```python
from build123d import *

# Parameters (mm, degrees)
F1_DEPTH  = 3.5
F2_W      = 30
F2_H      = 3
F3_DEPTH  = 14.5
F4_W      = 30
F4_H      = 3
F5_DEPTH  = 15
F6_W      = 3
F6_H      = 75
F7_DEPTH  = 14.5
F8_W      = 3
F8_H      = 75
F9_DEPTH  = 14.5
F10_W     = 3
F10_H     = 75
F11_DEPTH = 3
F12_W     = 3
F12_H     = 75
F13_DEPTH = 3
F14_R     = 2
F15_R     = 2
F16_R     = 2
F18_D     = 4.4


with BuildPart() as f1:
    # F0 (on Front) → F1 (new body)
    with BuildSketch(Plane.XZ):
        Polygon((15, 82.5), (-15, 82.5), (-15, 37.5), (-39, 37.5), (-39, -37.5), (-15, -37.5), (-15, -82.5), (15, -82.5), (15, -37.5), (39, -37.5), (39, 37.5), (15, 37.5), align=None)
    extrude(amount=F1_DEPTH)

    # F2 (on face) → F3 (join)
    with BuildSketch(Plane.XZ.offset(3.5)):
        with Locations((0, -81)):
            Rectangle(F2_W, F2_H)
    extrude(amount=F3_DEPTH)

    # F4 (on face) → F5 (join)
    with BuildSketch(Plane.XY.offset(-79.5)):
        with Locations((0, -16.5)):
            Rectangle(F4_W, F4_H)
    extrude(amount=F5_DEPTH)

    # F6 (on face) → F7 (join)
    with BuildSketch(Plane.XZ.offset(3.5)):
        with Locations((-37.5, 0)):
            Rectangle(F6_W, F6_H)
    extrude(amount=F7_DEPTH)

    # F8 (on face) → F9 (join)
    with BuildSketch(Plane.XZ.offset(3.5)):
        with Locations((37.5, 0)):
            Rectangle(F8_W, F8_H)
    extrude(amount=F9_DEPTH)

    # F10 (on face) → F11 (join)
    with BuildSketch(Plane.YZ.offset(-36)):
        with Locations((-16.5, 0)):
            Rectangle(F10_W, F10_H)
    extrude(amount=F11_DEPTH)

    # F12 (on face) → F13 (join)
    with BuildSketch(Plane(origin=(36, 0, 0), x_dir=(0, -1, 0), z_dir=(-1, 0, 0))):
        with Locations((16.5, 0)):
            Rectangle(F12_W, F12_H)
    extrude(amount=F13_DEPTH)

    # F14
    f14_edges = [f1.edges().sort_by_distance(p)[0] for p in [
        (39, -18, 0),
    ]]
    fillet(f14_edges, radius=F14_R)

    # F15
    f15_edges = [f1.edges().sort_by_distance(p)[0] for p in [
        (-39, -18, 0),
    ]]
    fillet(f15_edges, radius=F15_R)

    # F16
    f16_edges = [f1.edges().sort_by_distance(p)[0] for p in [
        (0, -18, -82.5),
    ]]
    fillet(f16_edges, radius=F16_R)

    # F18 (through all)
    with Locations(Plane.XZ.offset(3.5)):
        with Locations((0, 74.796483)):
            Hole(F18_D / 2)


solid = f1.part
```
Model file for the job. Use its own axes, mm. A direction names the side the tool comes from. Coordinates: 2 decimals unless noted, no trailing zeros. Write each loop counter-clockwise with the first axis right and the second up, starting at its lowest first coordinate (ties: lowest second). Pieces come first, ordered by that corner, then holes. Notation, with made-up numbers: (-39.5, 7.25) - (11.5, 7.25) arc R33 cw to (11.5, 43.25) - close; hole circle Ø6 at (6.25, 58.5). An arc over 180 degrees is marked (long way). Use a Markdown table: item, result. Add a question column.
Item 1: Band-saw the part on A-A, the plane x = 0. Write the cut outline in (y, z), and give its area (3 significant figures).
Item 2: Two-plate mould, pull along Y, no slides. Class faces 4 (the face through (-33, -17, 1)), 5 (the face through (-36, -9, -1)), 6 (the face through (-1, 0, 1)): pulls with the +Y half, pulls with the -Y half, needs draft (parallel to the pull), parting line crosses it, or undercut.
Item 3: Band-saw the part on C-C, the plane z = -26. Write the cut outline in (x, y), and give its area (3 significant figures).
Item 4: Drill centre lines: line 1 along Z through (x, y) = (0, -1.2); line 2 along X through (y, z) = (-9.5, 4.5); line 3 along Y through (x, z) = (35, 36). Where is each one in solid material? Low to high.
Item 5: Drop flat-ended pins along their axis: pin 1 (8 mm diameter, centred on x = -16, z = 52, fed in from -Y); pin 2 (5 mm diameter, centred on x = -6, y = -10.5, fed in from +Z); pin 3 (3 mm diameter, centred on y = -2, z = 61, fed in from -X). Give the stop position or say it passes through.
Item 6: 3-axis set-ups, long thin cutter, end or side, ignore diameter. For faces 1 (the face through (31, -3, 37.5)), 2 (the face through (15, -3, -65)), 3 (the face through (-15, -3, -65)): which of +Z, -Z, +X, -X, +Y, -Y reach the whole face in a straight line?
Item 7: Band-saw the part on B-B, the plane y = -12.75. Write the cut outline in (x, z).
Item 8: Band-saw the part on D-D, the plane x = -12. Write the cut outline in (y, z).
A:
| question | item | result |
|---|---|---|
| 1 | outline | (-18, -80.5) arc R2 ccw to (-16, -82.5) - (0, -82.5) - (0, 72.6) - (-3.5, 72.6) - (-3.5, -79.5) - (-15, -79.5) - (-15, -64.5) - (-18, -64.5) - close; (-3.5, 77) - (0, 77) - (0, 82.5) - (-3.5, 82.5) - close |
| 1 | area | 650 mm² |
| 2 | face 4 | needs draft |
| 2 | face 5 | undercut |
| 2 | face 6 | pulls with the +Y half |
| 3 | outline | (-39, -16) arc R2 ccw to (-37, -18) - (-33, -18) - (-33, -15) - (-36, -15) - (-36, -3.5) - (36, -3.5) - (36, -15) - (33, -15) - (33, -18) - (37, -18) arc R2 ccw to (39, -16) - (39, 0) - (-39, 0) - close |
| 3 | area | 376 mm² |
| 4 | line 1 | z = -82.5 to 72.6, 77 to 82.5 |
| 4 | line 2 | x = -39 to -36, 36 to 39 |
| 4 | line 3 | y = -18 to -15, -3.5 to 0 |
| 5 | pin 1 | stops at y = -3.5 |
| 5 | pin 2 | stops at z = -79.5 |
| 5 | pin 3 | stops at x = -15 |
| 6 | face 1 | +Z, +X, +Y, -Y |
| 6 | face 2 | -Z, +X, +Y, -Y |
| 6 | face 3 | -Z, -X, +Y, -Y |
| 7 | outline | (-39, -37.5) - (-36, -37.5) - (-36, 37.5) - (-39, 37.5) - close; (-15, -82.5) - (15, -82.5) - (15, -79.5) - (-15, -79.5) - close; (36, -37.5) - (39, -37.5) - (39, 37.5) - (36, 37.5) - close |
| 8 | outline | (-18, -80.5) arc R2 ccw to (-16, -82.5) - (0, -82.5) - (0, 82.5) - (-3.5, 82.5) - (-3.5, -79.5) - (-15, -79.5) - (-15, -64.5) - (-18, -64.5) - close |
